Check sheet for the modelled part. Datum: model origin and axes. Units: mm. A direction names the side the tool comes from. Coordinates: 2 decimals unless noted, no trailing zeros. Write each loop counter-clockwise with the first axis right and the second up, starting at its lowest first coordinate (ties: lowest second). Pieces come first, ordered by that corner, then holes. Notation, with made-up numbers: (52.25, 64) -> (61.25, 64) arc R23 cw to (61.25, 77) -> close; hole circle Ø1 at (7.5, -8). An arc over 180 degrees is marked (long way). One line per item, written item: value. Start each with the question number.
1) Gauge pin test, flat ends, axial feed: P1, Ø0.6, axis at x = 48, y = 6.5, coming from the +Z side; P2, Ø2.5, axis at y = 7.5, z = -4, coming from the +X side; P3, Ø10, axis at x = 8, y = 17.5, coming from the -Z side. Record the tip position at first contact, or that the pin passes through.
2) Scan lines: line 1 along Z through (x, y) = (2.5, 1) (3 decimals); line 2 along X through (y, z) = (16.25, 0); line 3 along X through (y, z) = (1.5, -8.25). Record each from-to range of solid material in increasing order. Write a range as [from, to].
3) Draft check along Z on faces 5 (the cylindrical face through (47.39, 3.55, -6.78)), 6 (the cylindrical face through (-49, 9, 8)), 7 (the cylindrical face through (-49, 9, -8)). Enter one of: +Z half, -Z half, draft (parallel to the pull), parting line (faces both ways), or undercut.
4) Sectioned sample at A-A on x = 24. Enter the section's corners in (y, z).
5) Set-up check for faces 1 (the flat face through (5, 15, 0)), 2 (the flat face through (-23, 20, 0)), 3 (the cylindrical face through (4.1, 15.03, -9.14)), 4 (the cylindrical face through (-47.859, 8.619, 7.797)): record each of +Z, -Z, +X, -X, +Y, -Y from which the full face is reachable in a straight line by a thin tool's end or side.
6) Sectioned sample at B-B on x = -22.5. Enter the section's corners in (y, z).
```python
from build123d import *

# Parameters (mm, degrees)
SKETCH1_W                    = 100
SKETCH1_H                    = 20
BOSS_EXTRUDE1_DEPTH          = 20
FILLET1_R                    = 5
FILLET2_R                    = 7.5
CUT_EXTRUDE1_DEPTH           = 58.445626465
CUT_EXTRUDE1_DEPTH_BACK      = 58.445626465
SKETCH3_W                    = 45
SKETCH3_H                    = 10
FILLET3_R                    = 3
SHELL1_T                     = -1
BOSS_EXTRUDE3_REACH          = 56.772
M1_2X0_25_TAPPED_HOLE2_D     = 0.95
M1_2X0_25_TAPPED_HOLE2_DEPTH = 3.65
M1_2X0_25_TAPPED_HOLE2_TIP   = 0.285408794
M3_TAPPED_HOLE1_D            = 2.5
M3_TAPPED_HOLE1_DEPTH        = 8.5
M3_TAPPED_HOLE1_TIP          = 0.751075774


with BuildPart() as part:
    # Sketch1 → Boss-Extrude1 (new body)
    with BuildSketch(Plane(origin=(0, 0, 0), x_dir=(1, 0, 0), z_dir=(0, 1, 0))):
        Rectangle(SKETCH1_W, SKETCH1_H)
    extrude(amount=BOSS_EXTRUDE1_DEPTH)

    # Fillet1
    fillet1_edges = [part.edges().sort_by_distance(p)[0] for p in [
        (-50, 10, 10),
        (-50, 10, -10),
    ]]
    fillet(fillet1_edges, radius=FILLET1_R)

    # Fillet2
    fillet2_edges = [part.edges().sort_by_distance(p)[0] for p in [
        (50, 10, 10),
        (50, 10, -10),
    ]]
    fillet(fillet2_edges, radius=FILLET2_R)

    # Sketch3 → Cut-Extrude1 (cut, two sides: drawn at the far end of the back side and taken through both)
    with BuildSketch(Plane.XY.offset(10).offset(-CUT_EXTRUDE1_DEPTH_BACK)):
        with Locations((27.5, 15)):
            Rectangle(SKETCH3_W, SKETCH3_H)
    extrude(amount=CUT_EXTRUDE1_DEPTH + CUT_EXTRUDE1_DEPTH_BACK, mode=Mode.SUBTRACT)

    # Fillet3
    fillet3_edges = [part.edges().sort_by_distance(p)[0] for p in [
        (-50, 20, 0),
        (-20, 20, 10),
        (-48.535533906, 20, 8.535533906),
        (-48.535533906, 20, -8.535533906),
        (47.803300859, 10, 7.803300859),
        (-20, 20, -10),
        (5, 10, 0),
        (5, 15, 10),
        (5, 15, -10),
        (5, 20, 0),
        (47.803300859, 10, -7.803300859),
        (50, 10, 0),
        (23.75, 10, 10),
        (23.75, 10, -10),
    ]]
    fillet(fillet3_edges, radius=FILLET3_R)

    # Shell1
    shell1_openings = [part.faces().sort_by_distance(p)[0] for p in [
        (-0.326782527, 0, 0),
    ]]
    offset(amount=SHELL1_T, openings=shell1_openings, kind=Kind.INTERSECTION)

    # Sketch4 → Boss-Extrude3 (add, up to next)
    with BuildSketch(Plane.XZ, mode=Mode.PRIVATE) as boss_extrude3_sk1:
        with BuildLine():
            Line((1.5, -7.5), (1.5, -9))
            Line((1.5, -9), (3.5, -9))
            Line((3.5, -9), (3.5, -7.5))
            ThreePointArc((3.5, -7.5), (2.5, -6.5), (1.5, -7.5))
        make_face()
    boss_extrude3_tool1 = extrude(boss_extrude3_sk1.sketch, amount=-BOSS_EXTRUDE3_REACH, mode=Mode.PRIVATE) - part.part
    # Sketch4 → Boss-Extrude3 (add, up to next)
    with BuildSketch(Plane.XZ, mode=Mode.PRIVATE) as boss_extrude3_sk2:
        with BuildLine():
            Line((1.5, 7.5), (1.5, 9))
            Line((1.5, 9), (3.5, 9))
            Line((3.5, 9), (3.5, 7.5))
            ThreePointArc((3.5, 7.5), (2.5, 6.5), (1.5, 7.5))
        make_face()
    boss_extrude3_tool2 = extrude(boss_extrude3_sk2.sketch, amount=-BOSS_EXTRUDE3_REACH, mode=Mode.PRIVATE) - part.part
    # Sketch4 → Boss-Extrude3 (add, up to next)
    with BuildSketch(Plane.XZ, mode=Mode.PRIVATE) as boss_extrude3_sk3:
        with BuildLine():
            Line((41.5, -7.5), (41.5, -9))
            Line((41.5, -9), (43.5, -9))
            Line((43.5, -9), (43.5, -7.5))
            ThreePointArc((43.5, -7.5), (42.5, -6.5), (41.5, -7.5))
        make_face()
    boss_extrude3_tool3 = extrude(boss_extrude3_sk3.sketch, amount=-BOSS_EXTRUDE3_REACH, mode=Mode.PRIVATE) - part.part
    # Sketch4 → Boss-Extrude3 (add, up to next)
    with BuildSketch(Plane.XZ, mode=Mode.PRIVATE) as boss_extrude3_sk4:
        with BuildLine():
            Line((41.5, 7.5), (41.5, 9))
            Line((41.5, 9), (43.5, 9))
            Line((43.5, 9), (43.5, 7.5))
            ThreePointArc((43.5, 7.5), (42.5, 6.5), (41.5, 7.5))
        make_face()
    boss_extrude3_tool4 = extrude(boss_extrude3_sk4.sketch, amount=-BOSS_EXTRUDE3_REACH, mode=Mode.PRIVATE) - part.part
    # Sketch4 → Boss-Extrude3 (add, up to next)
    with BuildSketch(Plane.XZ, mode=Mode.PRIVATE) as boss_extrude3_sk5:
        with BuildLine():
            Line((47, 2.431166482), (49, 2.431166482))
            Line((49, 2.431166482), (49, -1.568833518))
            Line((49, -1.568833518), (47, -1.568833518))
            ThreePointArc((47, -1.568833518), (45, 0.431166482), (47, 2.431166482))
        make_face()
    boss_extrude3_tool5 = extrude(boss_extrude3_sk5.sketch, amount=-BOSS_EXTRUDE3_REACH, mode=Mode.PRIVATE) - part.part
    # Sketch4 → Boss-Extrude3 (add, up to next)
    with BuildSketch(Plane.XZ, mode=Mode.PRIVATE) as boss_extrude3_sk6:
        with BuildLine():
            Line((-47, 2), (-49, 2))
            Line((-49, 2), (-49, -2))
            Line((-49, -2), (-47, -2))
            ThreePointArc((-47, -2), (-45, 0), (-47, 2))
        make_face()
    boss_extrude3_tool6 = extrude(boss_extrude3_sk6.sketch, amount=-BOSS_EXTRUDE3_REACH, mode=Mode.PRIVATE) - part.part
    add(boss_extrude3_tool1.solids().sort_by_distance((2.5, 0, -7.846402))[0])
    add(boss_extrude3_tool2.solids().sort_by_distance((2.5, 0, 7.846402))[0])
    add(boss_extrude3_tool3.solids().sort_by_distance((42.5, 0, -7.846402))[0])
    add(boss_extrude3_tool4.solids().sort_by_distance((42.5, 0, 7.846402))[0])
    add(boss_extrude3_tool5.solids().sort_by_distance((47.1867, 0, 0.431166))[0])
    add(boss_extrude3_tool6.solids().sort_by_distance((-47.1867, 0, 0))[0])

    # M1.2x0.25 Tapped Hole2
    with Locations(Plane(origin=(0, 0, 0), x_dir=(-1, 0, 0), z_dir=(0, -1, 0))):
        with Locations((-2.5, -7.5), (-2.5, 7.5), (-42.5, 7.5), (-42.5, -7.5)):
            Hole(M1_2X0_25_TAPPED_HOLE2_D / 2, depth=M1_2X0_25_TAPPED_HOLE2_DEPTH)
            with Locations((0, 0, -(M1_2X0_25_TAPPED_HOLE2_DEPTH + M1_2X0_25_TAPPED_HOLE2_TIP / 2))):  # 118° drill point
                Cone(0, M1_2X0_25_TAPPED_HOLE2_D / 2, M1_2X0_25_TAPPED_HOLE2_TIP, mode=Mode.SUBTRACT)

    # M3 Tapped Hole1
    with Locations(Plane(origin=(0, 0, 0), x_dir=(-1, 0, 0), z_dir=(0, -1, 0))):
        with Locations((-47, -0.431166482), (47, 0)):
            Hole(M3_TAPPED_HOLE1_D / 2, depth=M3_TAPPED_HOLE1_DEPTH)
            with Locations((0, 0, -(M3_TAPPED_HOLE1_DEPTH + M3_TAPPED_HOLE1_TIP / 2))):  # 118° drill point
                Cone(0, M3_TAPPED_HOLE1_D / 2, M3_TAPPED_HOLE1_TIP, mode=Mode.SUBTRACT)


solid = part.part
```
Answers:
1. P1: stops at z = 7.9
1. P2: stops at x = 49.99
1. P3: stops at z = -9.82
2. line 1: z = [-10, -7.975], [-7.025, -6.5], [6.5, 7.025], [7.975, 10]
2. line 2: x = [-50, -45], [4, 5]
2. line 3: x = [-48.8, -47.33], [1.5, 3.5], [41.5, 43.5], [45.53, 47.32]
3. face 5: undercut
3. face 6: +Z half
3. face 7: -Z half
4. outline: (0, -10) -> (7, -10) arc R3 ccw to (10, -7) -> (10, 7) arc R3 ccw to (7, 10) -> (0, 10) -> (0, 9) -> (7, 9) arc R2 cw to (9, 7) -> (9, -7) arc R2 cw to (7, -9) -> (0, -9) -> close
5. face 1: +Z, -Z, +X, +Y
5. face 2: +Z, -Z, +X, -X, +Y
5. face 3: -Z, +X, +Y
5. face 4: -Y
6. outline: (0, -10) -> (17, -10) arc R3 ccw to (20, -7) -> (20, 7) arc R3 ccw to (17, 10) -> (0, 10) -> (0, 9) -> (17, 9) arc R2 cw to (19, 7) -> (19, -7) arc R2 cw to (17, -9) -> (0, -9) -> close
